Design review of the part shown in the three views and the two pictorial views. Dimensions are in mm from the part's minimum x, y and z. A direction names the side the tool comes from. Coordinates: 2 decimals unless noted, no trailing zeros. Order: outer loops, then holes, each group sorted by start corner. A loop starts at its lowest first (then second) coordinate and runs counter-clockwise, first axis right, second up. Notation, with made-up numbers: (-10, 86.5) - (23, 86.5) arc R16 ccw to (23, 96.5) - close; hole circle Ø11 at (89, -6.75). An arc over 180 degrees is marked (long way). One line per item, written item: value. Start each with the question number.
(1) Mouldability with a two-part tool opening along X and no side actions: class the marked faces 1, 2 and 3 as released by +X, released by -X, zero draft, split by the parting line, or undercut.
(2) To check wall thickness, follow line 1 along X through (y, z) = (2.95, 1.55); line 2 along Y through (x, z) = (6.25, 0.5); line 3 along Z through (x, y) = (1.5, 3.15). State the ranges of each line that lie inside material, in increasing order.
(3) Clearance check with a flat-ended pin moving along its axis: pin 1 (0.7 mm diameter, centred on x = 0, y = 3, fed in from -Z). State where the tip first meets the part, or that it passes through.
(4) For the marked faces 4, 5 and 6, list the 3-axis set-ups (+Z, -Z, +X, -X, +Y, -Y) from which the entire face can be reached by the end or side of a thin tool; tool diameter is ignored.
(5) Consider section B-B on z = 1.95. Write out the cut boundary in (x, y).
(6) Consider section C-C on y = 1.75. Write out the cut boundary in (x, z).
(7) Consider section A-A on z = 0.4. Write out the cut boundary in (x, y).
(8) Consider section D-D on x = 3.75. Write out the cut boundary in (y, z).
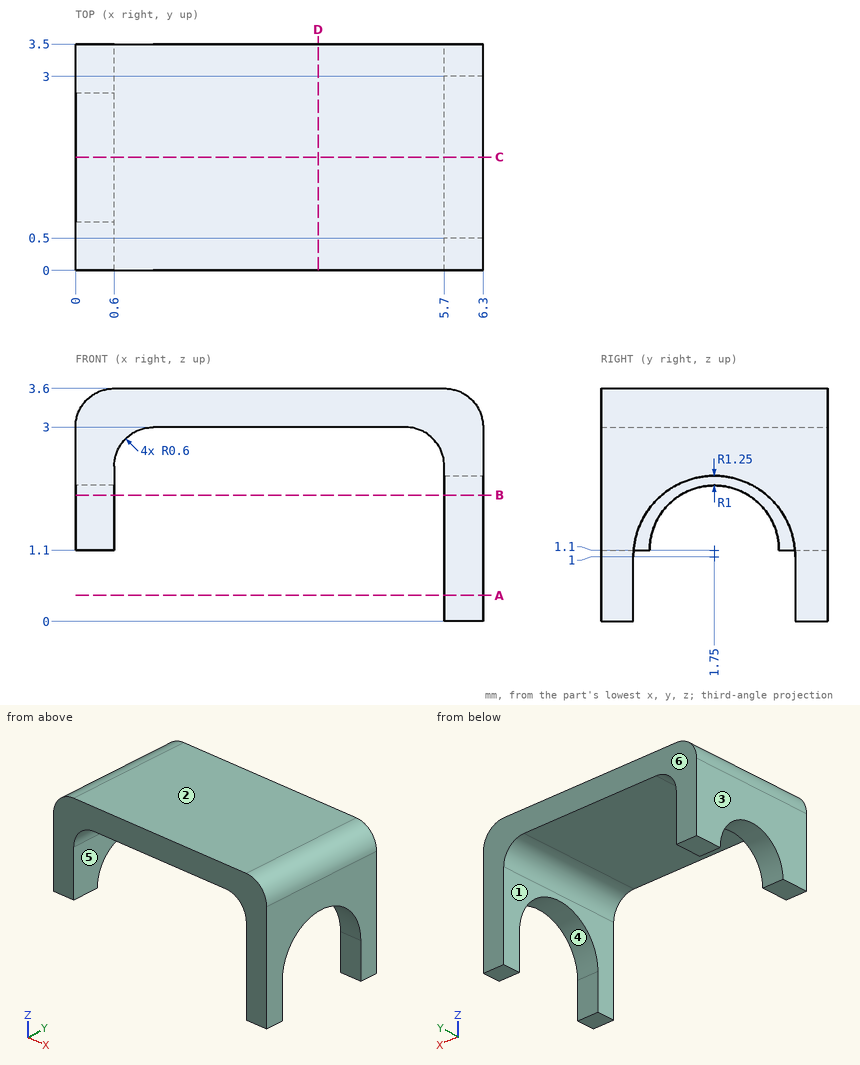
Geometry check:
1. face 1: undercut
1. face 2: zero draft
1. face 3: released by -X
2. line 1: x = 0 to 0.6, 5.7 to 6.3
2. line 2: y = 0 to 0.5, 3 to 3.5
2. line 3: z = 3 to 3.6
3. pin 1: stops at z = 1.1
4. face 4: -Z, +X
4. face 5: -Z, +Y, -Y
4. face 6: +Z, -Z, +X, -X, +Y
5. outline: (0, 0) - (0.6, 0) - (0.6, 1.22) - (0, 1.22) - close; (0, 2.28) - (0.6, 2.28) - (0.6, 3.5) - (0, 3.5) - close; (5.7, 0) - (6.3, 0) - (6.3, 0.94) - (5.7, 0.94) - close; (5.7, 2.56) - (6.3, 2.56) - (6.3, 3.5) - (5.7, 3.5) - close
6. outline: (0, 2.1) - (0.6, 2.1) - (0.6, 2.4) arc R0.6 cw to (1.2, 3) - (5.1, 3) arc R0.6 cw to (5.7, 2.4) - (5.7, 2.25) - (6.3, 2.25) - (6.3, 3) arc R0.6 ccw to (5.7, 3.6) - (0.6, 3.6) arc R0.6 ccw to (0, 3) - close
7. outline: (5.7, 0) - (6.3, 0) - (6.3, 0.5) - (5.7, 0.5) - close; (5.7, 3) - (6.3, 3) - (6.3, 3.5) - (5.7, 3.5) - close
8. outline: (0, 3) - (3.5, 3) - (3.5, 3.6) - (0, 3.6) - close
